Read the model definition and answer for the solid it produces. Units are mm, in the model's axes. A direction names the side the tool comes from. Give positions to 0.01 mm unless a question says otherwise; leave off trailing zeros. Order: outer loops, then holes, each group sorted by start corner. A loop starts at its lowest first (then second) coordinate and runs counter-clockwise, first axis right, second up. Notation, with made-up numbers: (7, 13) -> (55, 13) arc R21 ccw to (55, 39) -> close; hole circle Ø11 at (-6.75, 79.25). An arc over 180 degrees is marked (long way). Use one line per item in the form item = value.
```python
from build123d import *

# Parameters (mm, degrees)
SKETCH1_W              = 22.225
SKETCH1_H              = 22.225
BOSS_EXTRUDE1_DEPTH    = 25.4
SKETCH2_R              = 6.35
BOSS_EXTRUDE2_DEPTH    = 6.35
F_10_32_TAPPED_HOLE1_D = 4.0386
SKETCH6_W              = 17.145
SKETCH6_H              = 17.145
SKETCH6_R              = 5.1943
CUT_EXTRUDE1_DEPTH     = 21.59
SKETCH7_W              = 17.145
SKETCH7_H              = 17.145
SKETCH7_R              = 5.1943
BOSS_EXTRUDE3_DEPTH    = 3.81


with BuildPart() as part:
    # Sketch1 → Boss-Extrude1 (new body)
    with BuildSketch(Plane(origin=(0, 0, 0), x_dir=(1, 0, 0), z_dir=(0, 1, 0))):
        Rectangle(SKETCH1_W, SKETCH1_H)
    extrude(amount=BOSS_EXTRUDE1_DEPTH)

    # Sketch2 → Boss-Extrude2 (add)
    with BuildSketch(Plane(origin=(0, 25.4, 0), x_dir=(1, 0, 0), z_dir=(0, 1, 0))):
        with Locations(Location((0, 0, 0), (0, 0, 90))):
            Circle(SKETCH2_R)
    extrude(amount=BOSS_EXTRUDE2_DEPTH)

    # #10-32 Tapped Hole1 (through all)
    with Locations(Plane(origin=(0, 31.75, 0), x_dir=(1, 0, 0), z_dir=(0, 1, 0))):
        with Locations((0, 0)):
            Hole(F_10_32_TAPPED_HOLE1_D / 2)

    # Sketch6 → Cut-Extrude1 (cut)
    with BuildSketch(Plane.XZ):
        Rectangle(SKETCH6_W, SKETCH6_H)
        with Locations(Location((0, 0, 0), (0, 0, 270))):
            Circle(SKETCH6_R, mode=Mode.SUBTRACT)
    extrude(amount=-CUT_EXTRUDE1_DEPTH, mode=Mode.SUBTRACT)

    # Sketch7 → Boss-Extrude3 (add)
    with BuildSketch(Plane(origin=(0, 0, 0), x_dir=(-1, 0, 0), z_dir=(0, -1, 0))):
        Rectangle(SKETCH7_W, SKETCH7_H)
        with Locations(Location((0, 0, 0), (0, 0, 90))):
            Circle(SKETCH7_R, mode=Mode.SUBTRACT)
    extrude(amount=-BOSS_EXTRUDE3_DEPTH)


solid = part.part
```
Item 1: The part is cut by section A-A on x = 0. Give the vertices of the cut face in (y, z), and give its area (3 significant figures).
Checks:
outline = (0, -11.11) -> (25.4, -11.11) -> (25.4, -6.35) -> (31.75, -6.35) -> (31.75, -2.02) -> (0, -2.02) -> close; (0, 2.02) -> (31.75, 2.02) -> (31.75, 6.35) -> (25.4, 6.35) -> (25.4, 11.11) -> (0, 11.11) -> close; hole (3.81, -8.57) -> (21.59, -8.57) -> (21.59, -5.19) -> (3.81, -5.19) -> close; hole (3.81, 5.19) -> (21.59, 5.19) -> (21.59, 8.57) -> (3.81, 8.57) -> close
area = 397 mm²
Item 2: Determine the mould class of faces 1 (the flat face through (0, 13, -11.112)), 2 (the flat face through (0, 13, 8.572)), 3 (the flat face through (11.112, 13, 0)) for opening direction X: +X half, -X half, draft (parallel to the pull), parting line (faces both ways), or undercut.
Checks:
face_1 = draft
face_2 = undercut
face_3 = +X half
Item 3: The part is cut by section B-B on y = 19.5. Give the vertices of the cut face in (x, z), and give its area (3 significant figures).
Checks:
outline = (-11.11, -11.11) -> (11.11, -11.11) -> (11.11, 11.11) -> (-11.11, 11.11) -> close; circle Ø10.39 at (0, 0); hole (-8.57, -8.57) -> (8.57, -8.57) -> (8.57, 8.57) -> (-8.57, 8.57) -> close; hole circle Ø4.04 at (0, 0)
area = 272 mm²
Item 4: The part is cut by section C-C on z = 0. Give the vertices of the cut face in (x, y).
Checks:
outline = (-11.11, 0) -> (-2.02, 0) -> (-2.02, 31.75) -> (-6.35, 31.75) -> (-6.35, 25.4) -> (-11.11, 25.4) -> close; (2.02, 0) -> (11.11, 0) -> (11.11, 25.4) -> (6.35, 25.4) -> (6.35, 31.75) -> (2.02, 31.75) -> close; hole (-8.57, 3.81) -> (-5.19, 3.81) -> (-5.19, 21.59) -> (-8.57, 21.59) -> close; hole (5.19, 3.81) -> (8.57, 3.81) -> (8.57, 21.59) -> (5.19, 21.59) -> close
Item 5: Which of the six approach directions +Z, -Z, +X, -X, +Y, -Y give full straight-line access (tool end or side, diameter ignored) to faces 4 (the flat face through (0, 0, -3)), 5 (the cylindrical face through (3.86, 28.53, 5.04)), 6 (the flat face through (-8.572, 13, 0))?
Checks:
face_4 = +Z, -Z, +X, -X, -Y
face_5 = +Y
face_6 = none
Item 6: The part is cut by section D-D on x = 7.25. Give the vertices of the cut face in (y, z).
Checks:
outline = (0, -11.11) -> (25.4, -11.11) -> (25.4, 11.11) -> (0, 11.11) -> close; hole (3.81, -8.57) -> (21.59, -8.57) -> (21.59, 8.57) -> (3.81, 8.57) -> close
Item 7: Straight lines are drawn through the part: L1, parallel to X at y = 21, z = -7; L2, parallel to X at y = 20, z = -2.75; L3, parallel to Z at x = 0, y = 23.5. For each, find the intervals that lie inside material, in ascending order. Write a range as from..to.
Checks:
L1 = -11.11..-8.57, 8.57..11.11
L2 = -11.11..-8.57, -4.41..4.41, 8.57..11.11
L3 = -11.11..-2.02, 2.02..11.11
